Work out the finished part from the listing and answer in its coordinate system (mm). A direction names the side the tool comes from. Coordinates: 2 decimals unless noted, no trailing zeros. Loops run counter-clockwise (first coordinate to the right, second up) from the corner with the lowest first, then second, coordinate; pieces in that order, holes last. Notation, with made-up numbers: (84.25, -4.75) -> (142.25, -4.75) arc R12 ccw to (142.25, 0.25) -> close; hole circle Ø1 at (87, 68.25). An arc over 180 degrees is marked (long way). Answer as CSV lines item,"result".
```python
from build123d import *

# Parameters (mm, degrees)
CROQUIS1_W                   = 200
CROQUIS1_H                   = 110
CROQUIS1_W_2                 = 183
CROQUIS1_H_2                 = 93
CROQUIS1_W_3                 = 166.6
CROQUIS1_H_3                 = 8.2
CROQUIS1_H_4                 = 76.6
CROQUIS1_W_4                 = 8.2
SALIENTE_EXTRUIR1_DEPTH      = 2
CORTAR_EXTRUIR1_DEPTH        = 2
CROQUIS3_W                   = 200
CROQUIS3_H                   = 2
SALIENTE_EXTRUIR2_DEPTH      = 190
CROQUIS4_R                   = 4.35
CORTAR_EXTRUIR2_DEPTH        = 81
CROQUIS5_W                   = 250
CROQUIS5_H                   = 58
CROQUIS5_W_2                 = 200
CROQUIS5_W_3                 = 6
SALIENTE_EXTRUIR3_DEPTH      = 13
SALIENTE_EXTRUIR4_DEPTH      = 0.1
SALIENTE_EXTRUIR4_DEPTH_BACK = 56
CROQUIS7_R                   = 6
CORTAR_EXTRUIR3_DEPTH        = 80.1
CROQUIS10_W                  = 149.116642103
CROQUIS10_H                  = 58
SALIENTE_EXTRUIR5_DEPTH      = 10
CROQUIS11_W                  = 38
CROQUIS11_H                  = 21.5
CORTAR_EXTRUIR4_DEPTH        = 70


with BuildPart() as part:
    # Croquis1 → Saliente-Extruir1 (new body)
    # profile 1 of 6: a face of its own
    with BuildSketch(Plane(origin=(0, 0, 0), x_dir=(1, 0, 0), z_dir=(0, 1, 0))):
        Rectangle(CROQUIS1_W, CROQUIS1_H)
        Rectangle(CROQUIS1_W_2, CROQUIS1_H_2, mode=Mode.SUBTRACT)
    # profile 2 of 6: a face of its own
    with BuildSketch(Plane(origin=(0, 0, 0), x_dir=(1, 0, 0), z_dir=(0, 1, 0))):
        with Locations((0, 42.4)):
            Rectangle(CROQUIS1_W_3, CROQUIS1_H_3)
    # profile 3 of 6: a face of its own
    with BuildSketch(Plane(origin=(0, 0, 0), x_dir=(1, 0, 0), z_dir=(0, 1, 0))):
        Rectangle(CROQUIS1_W_3, CROQUIS1_H_4)
    # profile 4 of 6: a face of its own
    with BuildSketch(Plane(origin=(0, 0, 0), x_dir=(1, 0, 0), z_dir=(0, 1, 0))):
        with Locations((-87.4, 0)):
            Rectangle(CROQUIS1_W_4, CROQUIS1_H_4)
    # profile 5 of 6: a face of its own
    with BuildSketch(Plane(origin=(0, 0, 0), x_dir=(1, 0, 0), z_dir=(0, 1, 0))):
        with Locations((0, -42.4)):
            Rectangle(CROQUIS1_W_3, CROQUIS1_H_3)
    # profile 6 of 6: a face of its own
    with BuildSketch(Plane(origin=(0, 0, 0), x_dir=(1, 0, 0), z_dir=(0, 1, 0))):
        with Locations((87.4, 0)):
            Rectangle(CROQUIS1_W_4, CROQUIS1_H_4)
    extrude(amount=SALIENTE_EXTRUIR1_DEPTH)

    # Croquis2 → Cortar-Extruir1 (cut)
    with BuildSketch(Plane(origin=(0, 2, 0), x_dir=(1, 0, 0), z_dir=(0, 1, 0))):
        with BuildLine():
            ThreePointArc((-100, 47), (-97.656854249, 52.656854249), (-92, 55))
            Line((-92, 55), (-100, 55))
            Line((-100, 55), (-100, 47))
        make_face()
        with BuildLine():
            ThreePointArc((-92, -55), (-97.656854249, -52.656854249), (-100, -47))
            Line((-100, -47), (-100, -55))
            Line((-100, -55), (-92, -55))
        make_face()
        with BuildLine():
            Line((100, -55), (100, -47))
            ThreePointArc((100, -47), (97.656854249, -52.656854249), (92, -55))
            Line((92, -55), (100, -55))
        make_face()
        with BuildLine():
            Line((100, 55), (92, 55))
            ThreePointArc((92, 55), (97.656854249, 52.656854249), (100, 47))
            Line((100, 47), (100, 55))
        make_face()
    extrude(amount=-CORTAR_EXTRUIR1_DEPTH, mode=Mode.SUBTRACT)

    # Croquis3 → Saliente-Extruir2 (add)
    with BuildSketch(Plane(origin=(0, 2, 0), x_dir=(1, 0, 0), z_dir=(0, 1, 0))):
        with Locations((0, -30)):
            Rectangle(CROQUIS3_W, CROQUIS3_H)
        with Locations((0, 30)):
            Rectangle(CROQUIS3_W, CROQUIS3_H)
    extrude(amount=SALIENTE_EXTRUIR2_DEPTH)

    # Croquis4 → Cortar-Extruir2 (cut)
    with BuildSketch(Plane.XY.offset(31)):
        with BuildLine():
            ThreePointArc((-35.907198592, 185.411223689), (-27.45094246, 189.983179116), (-18.051821346, 192))
            Line((-18.051821346, 192), (-100, 192))
            Line((-100, 192), (-100, 73.004085605))
            ThreePointArc((-100, 73.004085605), (-82.293244846, 137.383897456), (-35.907198592, 185.411223689))
        make_face()
        with BuildLine():
            Line((12.058102776, 177.657452596), (98.130373638, 44.243495367))
            ThreePointArc((98.130373638, 44.243495367), (99.51807785, 41.83828614), (100, 39.103600519))
            Line((100, 39.103600519), (100, 192))
            Line((100, 192), (-13.35732151, 192))
            ThreePointArc((-13.35732151, 192), (0.971130931, 187.700726729), (12.058102776, 177.657452596))
        make_face()
        with Locations((35.02020603, 70.493592822)):
            Circle(CROQUIS4_R)
        with BuildLine():
            ThreePointArc((-28.192006816, 167.49912775), (-75.165619507, 106.707118451), (-73.438142939, 29.900839356))
            ThreePointArc((-73.438142939, 29.900839356), (-67.634394225, 27.289996416), (-65.023551285, 33.093745131))
            ThreePointArc((-65.023551285, 33.093745131), (-66.615983893, 103.895760975), (-23.31449202, 159.935408465))
            ThreePointArc((-23.31449202, 159.935408465), (-21.971389776, 166.156025506), (-28.192006816, 167.49912775))
        make_face()
    extrude(amount=-CORTAR_EXTRUIR2_DEPTH, mode=Mode.SUBTRACT)

    # Croquis5 → Saliente-Extruir3 (add)
    with BuildSketch(Plane(origin=(0, 2, 0), x_dir=(1, 0, 0), z_dir=(0, 1, 0))):
        with Locations((-225, 0)):
            Rectangle(CROQUIS5_W, CROQUIS5_H)
        Rectangle(CROQUIS5_W_2, CROQUIS5_H)
        with Locations((103, 0)):
            Rectangle(CROQUIS5_W_3, CROQUIS5_H)
    extrude(amount=SALIENTE_EXTRUIR3_DEPTH)

    # Croquis6 → Saliente-Extruir4 (add, two sides: drawn at the far end of the back side and taken through both)
    with BuildSketch(Plane.XY.offset(29).offset(-SALIENTE_EXTRUIR4_DEPTH_BACK)):
        with BuildLine():
            Line((-383.123851027, -103.888519267), (-135.216927507, -402.269059015))
            Line((-135.216927507, -402.269059015), (-120.435481517, -389.763884447))
            Line((-120.435481517, -389.763884447), (-362.287418648, -103.888519267))
            ThreePointArc((-362.287418648, -103.888519267), (-383.304553722, -47.792485784), (-350, 2))
            Line((-350, 2), (-350, 15))
            ThreePointArc((-350, 15), (-396.30683482, -36.156950221), (-383.123851027, -103.888519267))
        make_face()
    extrude(amount=SALIENTE_EXTRUIR4_DEPTH + SALIENTE_EXTRUIR4_DEPTH_BACK)

    # Croquis7 → Cortar-Extruir3 (cut)
    with BuildSketch(Plane(origin=(0, 0, -31), x_dir=(-1, 0, 0), z_dir=(0, 0, -1))):
        with Locations((0, 147)):
            Circle(CROQUIS7_R)
    extrude(amount=-CORTAR_EXTRUIR3_DEPTH, mode=Mode.SUBTRACT)

    # Croquis10 → Saliente-Extruir5 (add)
    with BuildSketch(Plane(origin=(0, 15, 0), x_dir=(1, 0, 0), z_dir=(0, 1, 0))):
        with Locations((31.441678948, 0)):
            Rectangle(CROQUIS10_W, CROQUIS10_H)
    extrude(amount=SALIENTE_EXTRUIR5_DEPTH)

    # Croquis11 → Cortar-Extruir4 (cut)
    with BuildSketch(Plane(origin=(106, 0, 0), x_dir=(0, 0, -1), z_dir=(1, 0, 0))):
        with Locations((0, 13.5)):
            Rectangle(CROQUIS11_W, CROQUIS11_H)
    extrude(amount=-CORTAR_EXTRUIR4_DEPTH, mode=Mode.SUBTRACT)


solid = part.part
```
(1) A cutting plane is placed at A-A, the plane x = -189. Write down the section's boundary in (y, z).
Computed values:
outline,"(-337.54, -27) -> (-308.72, -27) -> (-308.72, 29.1) -> (-337.54, 29.1) -> close; (2, -29) -> (15, -29) -> (15, 29) -> (2, 29) -> close"
(2) Which of the six approach directions +Z, -Z, +X, -X, +Y, -Y give full straight-line access (tool end or side, diameter ignored) to faces 5 (the face through (-1, 2, 43)), 6 (the face through (71, 2.75, 0)), 7 (the face through (-1, 0, -1)), 8 (the face through (-1, 2, -43))?
Computed values:
face 5,"+Z, +X, -X, +Y"
face 6,"+X"
face 7,"+Z, -Z, +X, -Y"
face 8,"-Z, +X, -X, +Y"
(3) A cutting plane is placed at C-C, the plane y = -345.5. Write down the section's boundary in (x, z), and give its area (3 significant figures).
Computed values:
outline,"(-182.38, -27) -> (-157.88, -27) -> (-157.88, 29.1) -> (-182.38, 29.1) -> close"
area,"1,370 mm2"
(4) Flat-ended cylindrical pins translate along their axes: pin 1 Ø19 at (x, y) = (0, 147) entering from +Z; pin 2 Ø1.6 at (y, z) = (1, -43) entering from -X; pin 3 Ø1 at (y, z) = (1, 43.5) entering from +X. Find the tip coordinate at first contact, or state that the pin passes through.
Computed values:
pin 1,"z = 31"
pin 2,"x = -100"
pin 3,"x = 100"
(5) A cutting plane is placed at B-B, the plane y = -197. Write down the section's boundary in (x, z), and give its area (3 significant figures).
Computed values:
outline,"(-305.76, -27) -> (-283.51, -27) -> (-283.51, 29.1) -> (-305.76, 29.1) -> close"
area,"1,250 mm2"
(6) Consider line 1 along Z through (x, y) = (46, 101.5); line 2 along Y through (x, z) = (0, 30); line 3 along Y through (x, z) = (-42.5, -14). Determine where each line is inside the solid, lowest interval first.
Computed values:
line 1,"-31 to -29, 29 to 31"
line 2,"0 to 141, 153 to 188.23"
line 3,"0 to 25"
(7) For a pull along X with two mould halves and no side action, classify faces 1 (the face through (-74.818, 107.747, 30.014)), 2 (the face through (-281, -208, -27)), 3 (the face through (-74.818, 107.747, -29.986)), 4 (the face through (-239.668, -248.827, 0.657)) as pulls with the +X half, pulls with the -X half, needs draft (parallel to the pull), parting line crosses it, or undercut.
Computed values:
face 1,"undercut"
face 2,"needs draft"
face 3,"undercut"
face 4,"pulls with the +X half"
